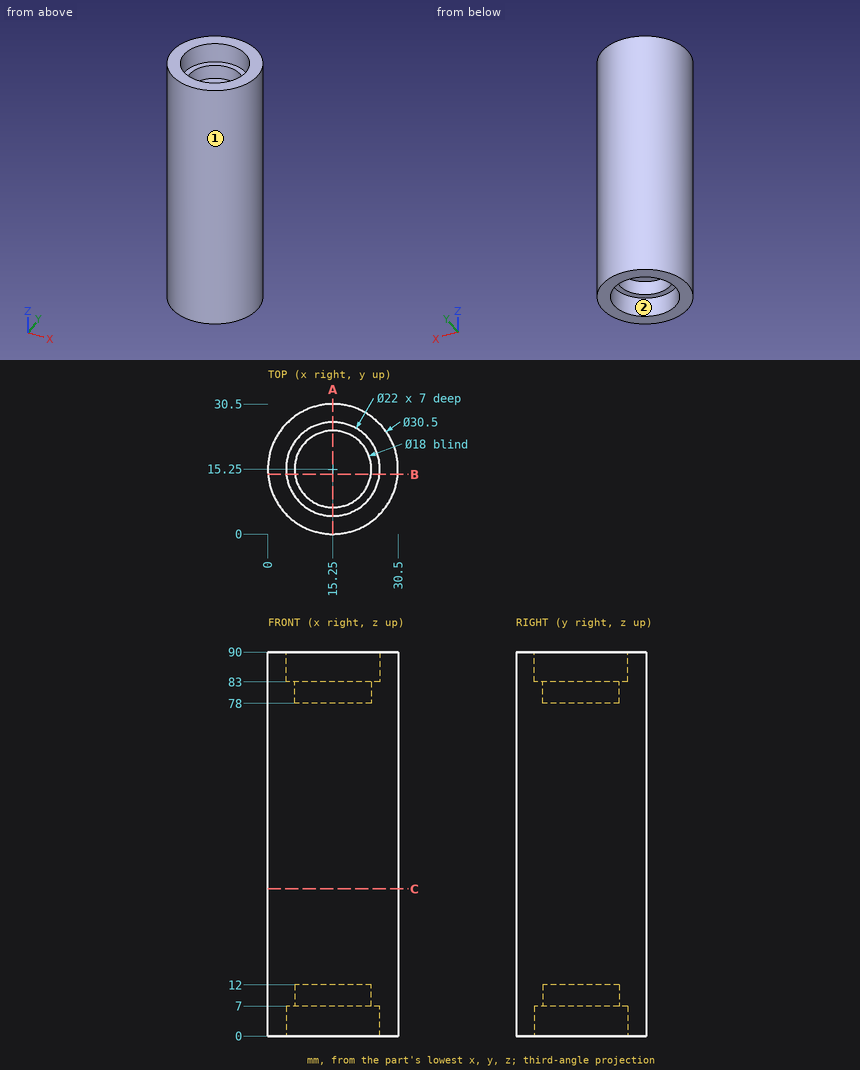
Part print with two shaded views. Sizes in mm from the minimum x, y, z corner. Coordinates: 2 decimals unless noted, no trailing zeros. Loops run counter-clockwise (first coordinate to the right, second up) from the corner with the lowest first, then second, coordinate; pieces in that order, holes last. Notation, with made-up numbers: M 66.5,70.5 L 73.5,70.5 A13 ccw 73.5,87.5 Z; hole C 83,40 d8. An arc over 180 degrees is marked long. Use CSV: the item, a comma, the result in double quotes. Start each with the question number.
1. Flat gauge pins, fed straight in: pin 1 (9 mm diameter, centred on x = 18.5, y = 11.5, fed in from +Z); pin 2 (14.5 mm diameter, centred on x = 15.25, y = 15.25, fed in from +Z); pin 3 (1.5 mm diameter, centred on y = 19, z = 25.5, fed in from -X). Where does each tip first touch, or does it go through?
2. Band-saw the part on A-A, the plane x = 15.25. List the corners of the cut face in (y, z).
3. Probe probe 1 along Y at (x, z) = (15, 9); probe 2 along Y at (x, z) = (15.25, 3). List the from-to ranges inside material, lowest first. Write a range as [from, to].
4. Band-saw the part on C-C, the plane z = 34.5. List the corners of the cut face in (x, y).
5. Two-plate mould, pull along Y, no slides. Class the marked faces 1 and 2: pulls with the +Y half, pulls with the -Y half, needs draft (parallel to the pull), parting line crosses it, or undercut.
6. Band-saw the part on B-B, the plane y = 14. List the corners of the cut face in (x, z).
Entries:
1,pin 1,"stops at z = 83"
1,pin 2,"stops at z = 78"
1,pin 3,"stops at x = 0.3"
2,outline,"M 0,0 L 4.25,0 L 4.25,7 L 6.25,7 L 6.25,12 L 24.25,12 L 24.25,7 L 26.25,7 L 26.25,0 L 30.5,0 L 30.5,90 L 26.25,90 L 26.25,83 L 24.25,83 L 24.25,78 L 6.25,78 L 6.25,83 L 4.25,83 L 4.25,90 L 0,90 Z"
3,probe 1,"y = [0, 6.25], [24.25, 30.5]"
3,probe 2,"y = [0, 4.25], [26.25, 30.5]"
4,outline,"C 15.25,15.25 d30.5"
5,face 1,"parting line crosses it"
5,face 2,"undercut"
6,outline,"M 0.05,0 L 4.32,0 L 4.32,7 L 6.34,7 L 6.34,12 L 24.16,12 L 24.16,7 L 26.18,7 L 26.18,0 L 30.45,0 L 30.45,90 L 26.18,90 L 26.18,83 L 24.16,83 L 24.16,78 L 6.34,78 L 6.34,83 L 4.32,83 L 4.32,90 L 0.05,90 Z"
